from build123d import *

# Parameters (mm, degrees)
SKETCH1_R           = 5
BOSS_EXTRUDE1_DEPTH = 5
BOSS_EXTRUDE2_DEPTH = 10
SKETCH3_W           = 12
SKETCH3_H           = 12
SKETCH3_W_2         = 10
SKETCH3_H_2         = 10
BOSS_EXTRUDE3_DEPTH = 12
SKETCH4_W           = 35
SKETCH4_H           = 35
BOSS_EXTRUDE4_DEPTH = 3
SKETCH5_R           = 10
BOSS_EXTRUDE5_DEPTH = 50
BOSS_EXTRUDE6_DEPTH = 5
FILLET1_R           = 10
FILLET4_R           = 5


with BuildPart() as part:
    # Sketch1 → Boss-Extrude1 (new body)
    with BuildSketch(Plane(origin=(0, 0, 0), x_dir=(1, 0, 0), z_dir=(0, 1, 0))):
        Polygon((0, 0), (0, 35), (35, 35), (35, 0), (35, -14), (21, -14), (21, 0), align=None)
        with Locations(Location((28, -7, 0), (0, 0, 270))):
            Circle(SKETCH1_R, mode=Mode.SUBTRACT)
        with BuildLine():
            Line((5.28246111, 33.217874153), (18.706396214, 18.392289297))
            ThreePointArc((18.706396214, 18.392289297), (18.531189995, 14.861099302), (15, 15.036305521))
            Line((15, 15.036305521), (1.576064896, 29.861890377))
            ThreePointArc((1.576064896, 29.861890377), (1.751271115, 33.393080372), (5.28246111, 33.217874153))
        make_face(mode=Mode.SUBTRACT)
    extrude(amount=BOSS_EXTRUDE1_DEPTH)

    # Sketch2 → Boss-Extrude2 (add)
    with BuildSketch(Plane.XZ):
        Polygon((30, -5), (20, -5), (20, 0), (35, 0), (35, -15), (30, -15), align=None)
    extrude(amount=BOSS_EXTRUDE2_DEPTH)

    # Sketch3 → Boss-Extrude3 (add)
    with BuildSketch(Plane(origin=(0, 5, 0), x_dir=(1, 0, 0), z_dir=(0, 1, 0))):
        with Locations((6, 6)):
            Rectangle(SKETCH3_W, SKETCH3_H)
        with Locations((30, 30)):
            Rectangle(SKETCH3_W_2, SKETCH3_H_2)
    extrude(amount=BOSS_EXTRUDE3_DEPTH)

    # Sketch4 → Boss-Extrude4 (add)
    with BuildSketch(Plane(origin=(0, 17, 0), x_dir=(1, 0, 0), z_dir=(0, 1, 0))):
        with Locations((17.5, 17.5)):
            Rectangle(SKETCH4_W, SKETCH4_H)
    extrude(amount=BOSS_EXTRUDE4_DEPTH)

    # Sketch5 → Boss-Extrude5 (add)
    with BuildSketch(Plane(origin=(0, 20, 0), x_dir=(1, 0, 0), z_dir=(0, 1, 0))):
        with Locations(Location((17.5, 17.5, 0), (0, 0, 270))):
            Circle(SKETCH5_R)
    extrude(amount=BOSS_EXTRUDE5_DEPTH)

    # Sketch6 → Boss-Extrude6 (add)
    with BuildSketch(Plane(origin=(0, 70, 0), x_dir=(1, 0, 0), z_dir=(0, 1, 0))):
        with BuildLine():
            Line((7.5, 17.5), (7.5, -32.5))
            Line((7.5, -32.5), (27.5, -32.5))
            Line((27.5, -32.5), (27.5, 17.5))
            ThreePointArc((27.5, 17.5), (17.5, 27.5), (7.5, 17.5))
        make_face()
    extrude(amount=BOSS_EXTRUDE6_DEPTH)

    # Fillet1
    # the kernel refuses this fillet: 10 mm, written as the material it adds along each edge
    with BuildSketch(Plane(origin=(21, 0, 0), x_dir=(-1, 0, 0), z_dir=(0, 1, 0))) as fillet1_piece_1:
        with BuildLine():
            CenterArc((FILLET1_R, FILLET1_R), FILLET1_R, 180, 90)
            Line((0, FILLET1_R), (0, 0))
            Line((0, 0), (FILLET1_R, 0))
        make_face()
    extrude(amount=5)

    # Fillet4
    fillet4_edges = [part.edges().sort_by_distance(p)[0] for p in [
        (35, 2.5, 14),
        (21, 2.5, 14),
    ]]
    fillet(fillet4_edges, radius=FILLET4_R)


solid = part.part
Read the model definition and answer for the solid it produces. Units are mm, in the model's axes. A direction names the side the tool comes from. Round coordinates to 2 decimals unless told otherwise and drop trailing zeros. Order: outer loops, then holes, each group sorted by start corner. A loop starts at its lowest first (then second) coordinate and runs counter-clockwise, first axis right, second up.
1) The part is cut by section A-A on x = 17.5. Write down the section's boundary in (y, z).
2) The part is cut by section D-D on y = 57. Write down the section's boundary in (x, z), plus the area to 3 significant figures.
3) For faces 1 (the face through (8.38, 2.46, -22.35)), 2 (the face through (30, 11, -25)), 3 (the face through (17.94, 47.11, -27.49)), determine the directions among +Z, -Z, +X, -X, +Y, -Y from which every point of the face is accessible in a straight line to the end or side of a thin tool.
4) The mould has two halves that part along Y. Classify faces 4 (the face through (1.711, 2.465, -33.356)), 5 (the face through (9, 12, 0)), 6 (the face through (17, 75, 2)): released by +Y, released by -Y, zero draft, split by the parting line, or undercut.
5) Flat-ended cylindrical pins translate along their axes: pin 1 (1 mm diameter, centred on x = 25, y = 46, fed in from -Z); pin 2 (1.5 mm diameter, centred on y = 72, z = -3, fed in from -X); pin 3 (10 mm diameter, centred on x = 21, z = -9.5, fed in from -Y); pin 4 (11 mm diameter, centred on x = 30.5, y = -4.5, fed in from +Z). Find the tip coordinate at first contact, or state that the pin passes through.
6) The part is cut by section B-B on z = 5.5. Write down the section's boundary in (x, y).
7) The part is cut by section C-C on x = 4. Write down the section's boundary in (y, z).
8) Straight lines are drawn through the part: L1, parallel to Y at x = 6, z = -19.5; L2, parallel to Y at x = 19, z = -6; L3, parallel to Y at x = 13, z = 27.5. For each, find the intervals that lie inside material, in ascending order.
Resolved:
1. outline: (0, -35) - (5, -35) - (5, -19.72) - (0, -19.72) - close; (0, -14.3) - (5, -14.3) - (5, 2.4) - (0, 2.4) - close; (17, -35) - (20, -35) - (20, -27.5) - (75, -27.5) - (75, 32.5) - (70, 32.5) - (70, -7.5) - (20, -7.5) - (20, 0) - (17, 0) - close
2. outline: circle Ø20 at (17.5, -17.5)
2. area: 314 mm2
3. face 1: -Y
3. face 2: +Z, +X, -X
3. face 3: none
4. face 4: zero draft
4. face 5: undercut
4. face 6: released by +Y
5. pin 1: stops at z = -24.64
5. pin 2: stops at x = 7.5
5. pin 3: stops at y = -10
5. pin 4: stops at z = 14
6. outline: (7.5, 70) - (27.5, 70) - (27.5, 75) - (7.5, 75) - close; (19.93, 0) - (23.23, 0) - (23.23, 5) - (19.93, 5) - close; (32.77, 0) - (35, 0) - (35, 5) - (32.77, 5) - close
7. outline: (0, -35) - (5, -35) - (5, -33.97) - (0, -33.97) - close; (0, -27.18) - (5, -27.18) - (5, -12) - (17, -12) - (17, -35) - (20, -35) - (20, 0) - (0, 0) - close
8. L1: y = 0 to 5, 17 to 20
8. L2: y = 0 to 5, 17 to 20, 70 to 75
8. L3: y = 70 to 75
